Could you check a few things on this model? Use its own coordinates, in mm. A direction names the side the tool comes from. Coordinates: 2 decimals unless noted, no trailing zeros. Write each loop counter-clockwise with the first axis right and the second up, starting at its lowest first coordinate (ties: lowest second). Pieces come first, ordered by that corner, then holes. Notation, with made-up numbers: M 81.5,25 L 116.5,25 A27 ccw 116.5,54 Z; hole C 22.25,71.25 d6. An arc over 180 degrees is marked long. Answer as CSV lines item,"result". Start each with the question number.
Item 1: Suppose I cut it at C-C, the plane y = 18.5. Write out the boundary of the cut face in (x, z).
Item 2: On a 3-axis mill with a long thin cutter (end or side, diameter ignored), from which of +Z, -Z, +X, -X, +Y, -Y can I reach the whole of each face in a straight line? I mean faces 1 (the flat face through (-2, 15, -10)), 2 (the flat face through (9, 15, -5)), 3 (the flat face through (10, 15, 3)). Say none if no direction works.
Item 3: We'd pull the mould along X, two halves only. Please class faces 4 (the cylindrical face through (-2.309, 7.395, -10.755)), 5 (the flat face through (-6.1, 15, -8.4)): +X half, -X half, draft (parallel to the pull), parting line (faces both ways), or undercut.
Item 4: Suppose I cut it at A-A, the plane x = 0. Write out the boundary of the cut face in (y, z), and give its area (4 significant figures).
Item 5: Suppose I cut it at B-B, the plane y = 36. Write out the boundary of the cut face in (x, z), and give its area (3 significant figures).
Item 6: I'm going to push flat-ended pins straight in: P1, Ø1.5, axis at x = 10, z = 3, coming from the +Y side; P2, Ø4, axis at x = -3, y = 24.5, coming from the -Z side; P3, Ø1.5, axis at x = 5.5, y = 24, coming from the +Z side. Where does each tip first touch, or does it pass through?
Item 7: If I drill on line 1 along Y through (x, z) = (-8.5, -7.5); line 2 along Y through (x, z) = (-6.5, -8.75); line 3 along X through (y, z) = (14, 0.5), over which ranges is the centre line in solid material (lowest first)? Write a range as [from, to].
```python
from build123d import *

# Parameters (mm, degrees)
SKETCH3_R           = 1
BOSS_EXTRUDE1_DEPTH = 15
CIRPATTERN1_COUNT   = 15
CHAMFER1_SIZE       = 0.5


with BuildPart() as part:
    # Sketch2 → Revolve1 (revolve)
    with BuildSketch(Plane(origin=(0, 0, 0), x_dir=(0, 0, -1), z_dir=(1, 0, 0)), mode=Mode.PRIVATE) as revolve1_sk:
        Polygon((0, 0), (10, 0), (10, 20), (14, 20), (14, 25), (7.5, 25), (7.5, 45), (0, 45), align=None)
    revolve(revolve1_sk.sketch.rotate(Axis((0, 45, 0), (0, -1, 0)), 180), axis=Axis((0, 45, 0), (0, -1, 0)))

    # Sketch3 → Boss-Extrude1 (add)
    with BuildSketch(Plane.XZ):
        with Locations((0, 10)):
            Circle(SKETCH3_R)
    boss_extrude1 = extrude(amount=-BOSS_EXTRUDE1_DEPTH)

    # CirPattern1: Boss-Extrude1 ×15 about axis
    cirpattern1_axis = Axis((0, 0, 0), (0, 1, 0))
    for i in range(1, CIRPATTERN1_COUNT):
        add(boss_extrude1.rotate(cirpattern1_axis, i * 360 / CIRPATTERN1_COUNT))

    # Chamfer1
    chamfer1_edges = [part.edges().sort_by_distance(p)[0] for p in [
        (0, 25, -14),
        (0, 20, -14),
    ]]
    chamfer(chamfer1_edges, length=CHAMFER1_SIZE)


solid = part.part
```
Ans:
1,outline,"C 0,0 d20"
2,face 1,"-Z, -X"
2,face 2,"-Z, +X"
2,face 3,"+Z, +X"
3,face 4,"undercut"
3,face 5,"draft"
4,outline,"M 0,-10 L 20,-10 L 20,-13.5 L 20.5,-14 L 24.5,-14 L 25,-13.5 L 25,-7.5 L 45,-7.5 L 45,7.5 L 25,7.5 L 25,13.5 L 24.5,14 L 20.5,14 L 20,13.5 L 20,10 L 15,10 L 15,11 L 0,11 Z"
4,area,"854.5 mm^2"
5,outline,"C 0,0 d15"
5,area,"177 mm^2"
6,P1,"stops at y = 25"
6,P2,"stops at z = -13.96"
6,P3,"stops at z = 13.17"
7,line 1,"y = [20, 25]"
7,line 2,"y = [0, 15], [20, 25]"
7,line 3,"x = [-9.99, 9.99]"
